```python
from build123d import *

# Parameters (mm, degrees)
SKETCH_W    = 18
SKETCH_H    = 80
PAD_DEPTH   = 1.6
FILLET_R    = 1.5
FILLET001_R = 1.5
FILLET002_R = 1.5
FILLET003_R = 1.5


with BuildPart() as part:
    # Sketch → Pad (new body)
    with BuildSketch(Plane.XY):
        with Locations((9, 40)):
            Rectangle(SKETCH_W, SKETCH_H)
    extrude(amount=PAD_DEPTH)

    # Fillet
    fillet_edges = [part.edges().sort_by_distance(p)[0] for p in [
        (0, 40, 1.6),
    ]]
    fillet(fillet_edges, radius=FILLET_R)

    # Fillet001
    fillet001_edges = [part.edges().sort_by_distance(p)[0] for p in [
        (9.75, 80, 1.6),
    ]]
    fillet(fillet001_edges, radius=FILLET001_R)

    # Fillet002
    fillet002_edges = [part.edges().sort_by_distance(p)[0] for p in [
        (18, 39.25, 1.6),
    ]]
    fillet(fillet002_edges, radius=FILLET002_R)

    # Fillet003
    fillet003_edges = [part.edges().sort_by_distance(p)[0] for p in [
        (9, 0, 1.6),
    ]]
    fillet(fillet003_edges, radius=FILLET003_R)


solid = part.part
```
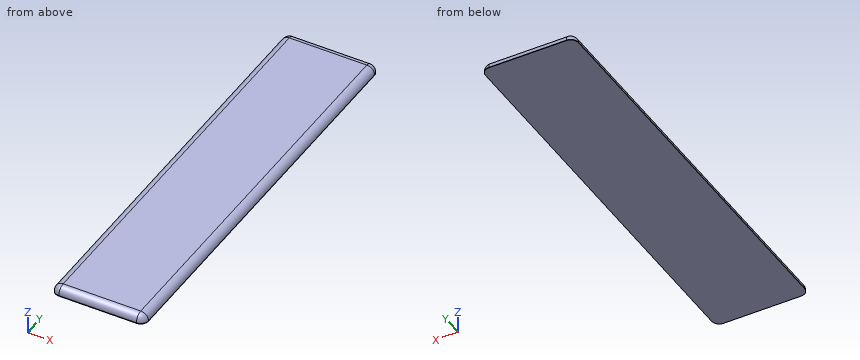
Geometry check sheet. Reference: the model listing, model coordinates, mm. Round coordinates to 2 decimals unless told otherwise and drop trailing zeros. Order: outer loops, then holes, each group sorted by start corner. A loop starts at its lowest first (then second) coordinate and runs counter-clockwise, first axis right, second up. Notation, with made-up numbers: (46.5, 6.25) -> (54.5, 6.25) arc R12 cw to (54.5, 15.25) -> close; hole circle Ø10 at (83.25, 37). An arc over 180 degrees is marked (long way). Return JSON: item names as keys, results as strings. Group by question number.
Q1. Material ranges on probe 1 along X at (y, z) = (59, 0.2); probe 2 along Y at (x, z) = (5, 0.3); probe 3 along X at (y, z) = (42, 0.5), recorded low to high. Write a range as from..to.
Q2. Section check A-A, the plane y = 67. Record the boundary of the cut face in (x, z), plus the area to 3 significant figures.
Q3. Section check B-B, the plane z = 0.85. Record the boundary of the cut face in (x, y).
Numbers:
{
 "1": {"probe 1": "0..18", "probe 2": "0.01..79.99", "probe 3": "0.05..17.95"},
 "2": {"outline": "(0, 0) -> (18, 0) -> (18, 0.1) arc R1.5 ccw to (16.5, 1.6) -> (1.5, 1.6) arc R1.5 ccw to (0, 0.1) -> close", "area": "27.8 mm^2"},
 "3": {"outline": "(0.2, 1.5) arc R1.3 ccw to (1.5, 0.2) -> (16.5, 0.2) arc R1.3 ccw to (17.8, 1.5) -> (17.8, 78.5) arc R1.3 ccw to (16.5, 79.8) -> (1.5, 79.8) arc R1.3 ccw to (0.2, 78.5) -> close"}
}
